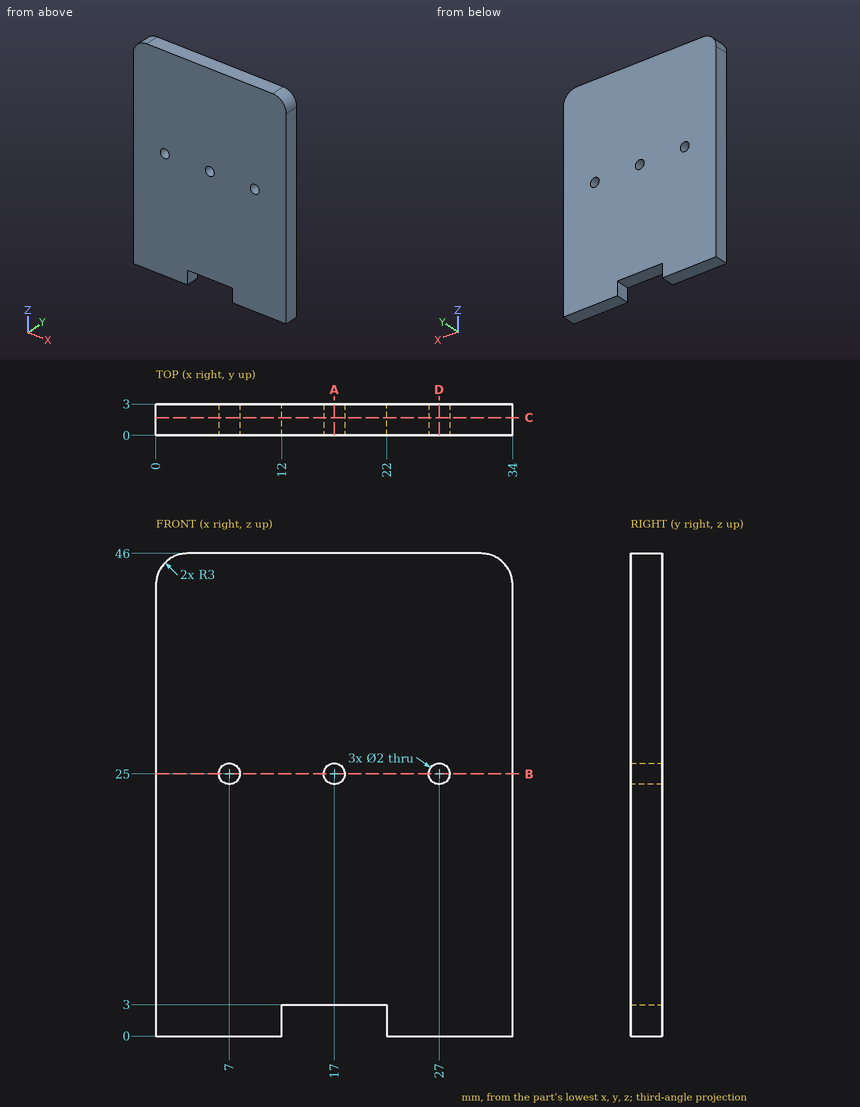
Design review of the part shown in the three views and the two pictorial views. Dimensions are in mm from the part's minimum x, y and z. Coordinates: 2 decimals unless noted, no trailing zeros. Order: outer loops, then holes, each group sorted by start corner. A loop starts at its lowest first (then second) coordinate and runs counter-clockwise, first axis right, second up. Notation, with made-up numbers: (-34.75, 84.25) - (-10.75, 84.25) arc R18 ccw to (-10.75, 109.25) - close; hole circle Ø10 at (56.5, 15.5). An arc over 180 degrees is marked (long way). Answer as CSV lines item,"result". Start each with the question number.
1) To check wall thickness, follow line 1 along X through (y, z) = (0.75, 25); line 2 along Z through (x, y) = (7, 1.2); line 3 along Z through (x, y) = (12.5, 0.85). State the ranges of each line that lie inside material, in increasing order. Write a range as [from, to].
2) Add section A-A (x = 17). State the section outline as (y, z) points, then the cut area to 3 significant figures.
3) Add section B-B (z = 25). State the section outline as (x, y) points, then the cut area to 3 significant figures.
4) Add section C-C (y = 1.7). State the section outline as (x, z) points, then the cut area to 3 significant figures.
5) Insertion check: P1, Ø1.5, axis at x = 14.5, y = 1, coming from the -Z side. The pin has a flat end and moves straight along its axis. Give the tip position at first contact, or say it passes through.
6) Add section D-D (x = 27). State the section outline as (y, z) points.
Result:
1,line 1,"[0, 6], [8, 16], [18, 26], [28, 34]"
1,line 2,"[0, 24], [26, 46]"
1,line 3,"[3, 46]"
2,outline,"(0, 3) - (3, 3) - (3, 24) - (0, 24) - close; (0, 26) - (3, 26) - (3, 46) - (0, 46) - close"
2,area,"123 mm^2"
3,outline,"(0, 0) - (6, 0) - (6, 3) - (0, 3) - close; (8, 0) - (16, 0) - (16, 3) - (8, 3) - close; (18, 0) - (26, 0) - (26, 3) - (18, 3) - close; (28, 0) - (34, 0) - (34, 3) - (28, 3) - close"
3,area,"84.0 mm^2"
4,outline,"(0, 0) - (12, 0) - (12, 3) - (22, 3) - (22, 0) - (34, 0) - (34, 43) arc R3 ccw to (31, 46) - (3, 46) arc R3 ccw to (0, 43) - close; hole circle Ø2 at (7, 25); hole circle Ø2 at (17, 25); hole circle Ø2 at (27, 25)"
4,area,"1,520 mm^2"
5,P1,"z = 3"
6,outline,"(0, 0) - (3, 0) - (3, 24) - (0, 24) - close; (0, 26) - (3, 26) - (3, 46) - (0, 46) - close"
